The drawing under review shows one solid part. Ordinate dimensions are in mm from its lowest x, y, z. Give positions to 0.01 mm unless a question says otherwise; leave off trailing zeros. Write each loop counter-clockwise with the first axis right and the second up, starting at its lowest first coordinate (ties: lowest second). Pieces come first, ordered by that corner, then holes. Notation, with made-up numbers: (-5.5, 20.5) - (25.5, 20.5) arc R17 cw to (25.5, 43.5) - close; hole circle Ø9 at (84.25, 40). An arc over 180 degrees is marked (long way). Write each question's results on one line, items separated by ' | '. Start each with the question number.
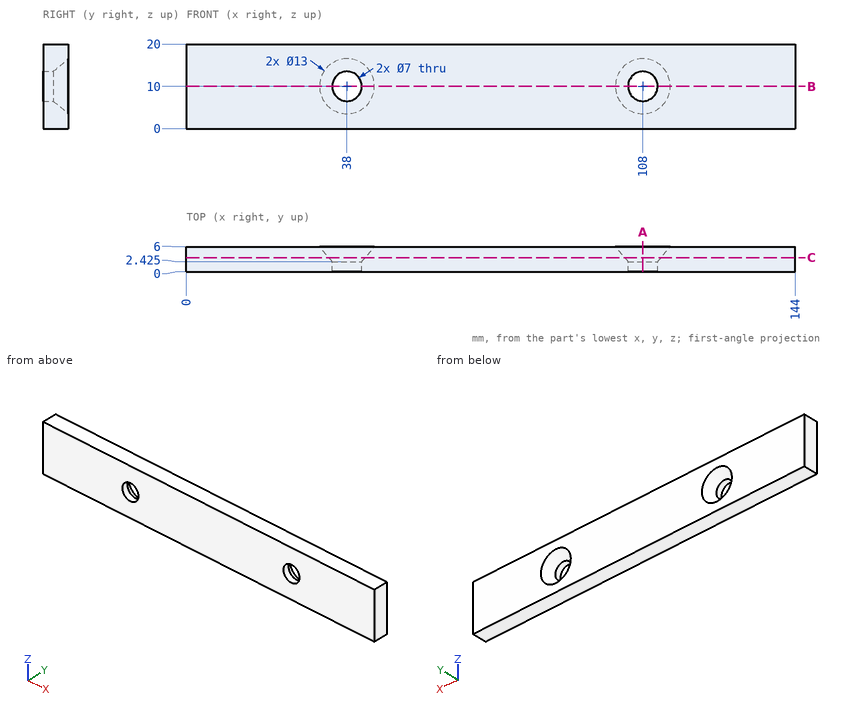
Q1. Add section C-C on y = 3.4. State the section outline as (x, z) points.
Q2. Add section B-B on z = 10. State the section outline as (x, y) points (1 decimal).
Q3. For line 1 along X through (y, z) = (1.5, 10); line 2 along Z through (x, y) = (38, 1.35); line 3 along X through (y, z) = (5.3, 9.25) (1 decimal), list the stretches that pass through material, from the lowest coordinate up. Write a range as [from, to].
Q4. Add section A-A on x = 108. State the section outline as (y, z) points (1 decimal).
Q5. Insertion check: P1, Ø5.5, axis at x = 108, z = 10, coming from the +Y side. The pin has a flat end and moves straight along its axis. Give the tip position at first contact, or say it passes through.
Result:
1) outline: (0, 0) - (144, 0) - (144, 20) - (0, 20) - close; hole circle Ø8.64 at (38, 10); hole circle Ø8.64 at (108, 10)
2) outline: (0, 0) - (34.5, 0) - (34.5, 2.4) - (31.5, 6) - (0, 6) - close; (41.5, 0) - (104.5, 0) - (104.5, 2.4) - (101.5, 6) - (44.5, 6) - (41.5, 2.4) - close; (111.5, 0) - (144, 0) - (144, 6) - (114.5, 6) - (111.5, 2.4) - close
3) line 1: x = [0, 34.5], [41.5, 104.5], [111.5, 144] | line 2: z = [0, 6.5], [13.5, 20] | line 3: x = [0, 32.1], [43.9, 102.1], [113.9, 144]
4) outline: (0, 0) - (6, 0) - (6, 3.5) - (2.4, 6.5) - (0, 6.5) - close; (0, 13.5) - (2.4, 13.5) - (6, 16.5) - (6, 20) - (0, 20) - close
5) P1: passes through
